The listing builds one solid part. Answer for the finished solid, in the listing's coordinates (mm). Face numbers are marked on the shaded views. A direction names the side the tool comes from. Coordinates: 2 decimals unless noted, no trailing zeros. Order: outer loops, then holes, each group sorted by start corner. A loop starts at its lowest first (then second) coordinate and runs counter-clockwise, first axis right, second up. Notation, with made-up numbers: (2, 42) -> (17, 42) arc R9 cw to (17, 50) -> close; hole circle Ø10 at (84, 17). An arc over 180 degrees is marked (long way). Write each question's results on one line, items separated by ' | '. Start each with the question number.
(1) Determine the mould class of the marked faces 1, 2 and 3 for opening direction X: +X half, -X half, draft (parallel to the pull), parting line (faces both ways), or undercut.
(2) The part is cut by section C-C, the plane z = -9. Count the separate pieces of the cut face and the enclosed holes in it, then the cut area to 3 significant figures.
(3) The part is cut by section B-B, the plane y = 9. Give the vertices of the cut face in (x, z), then the cut area to 3 significant figures.
(4) A tool of negligible diameter and unlimited length cuts with its end or side. For the marked faces 4 and 5, from which of +Z, -Z, +X, -X, +Y, -Y can it reach the whole face along a straight path? Write none if from no direction.
(5) The part is cut by section A-A, the plane x = 22. Give the vertices of the cut face in (y, z), then the cut area to 3 significant figures.
(6) Given pin 1 (10.5 mm diameter, centred on x = -37.69, z = 28.7, fed in from -Y); pin 2 (10.5 mm diameter, centred on x = -29.22, z = -27.5, fed in from +Y); pin 3 (5 mm diameter, centred on x = 9.56, z = 19.57, fed in from -Y); pin 4 (0.6 mm diameter, centred on x = -48, y = 7, fed in from +Z), each flat-ended and moving along its own axis, determine where each tip first touches the part or whether it passes through.
(7) Straight lines are drawn through the part: L1, parallel to X at y = 8.25, z = 23; L2, parallel to Y at x = 26.5, z = -26. For each, find the intervals that lie inside material, in ascending order.
```python
from build123d import *

# Parameters (mm, degrees)
SKETCH1_W               = 76.9234
SKETCH1_H               = 67.5
BASE_FLANGE1_DEPTH      = 0.7366
EDGE_FLANGE1_DEPTH      = 67.5
EDGE_FLANGE1_BEND_DEPTH = 67.5
CUT_EXTRUDE1_DEPTH      = 89.757105022
FILLET1_R               = 10
SKETCH14_R              = 4
CUT_EXTRUDE2_DEPTH      = 10


# Sheet-metal steps are written as plain solids
with BuildPart() as part:
    # Sketch1 → Base-Flange1 (new body)
    with BuildSketch(Plane(origin=(0, 0, 0), x_dir=(1, 0, 0), z_dir=(0, 1, 0))):
        with Locations((-8.2804, -1.046060421)):
            Rectangle(SKETCH1_W, SKETCH1_H)
    extrude(amount=-BASE_FLANGE1_DEPTH)

    # Edge-Flange1 section (across the edge) → Edge-Flange1 (add)
    with BuildSketch(Plane(origin=(31.1813, 0, 34.796060421), x_dir=(-1, 0, 0), z_dir=(0, 0, -1))):
        with BuildLine():
            Line((-0.7366, 0.7366), (-0.7366, 14.2634))
            Line((-0.7366, 14.2634), (0, 14.2634))
            Line((0, 14.2634), (0, 0.7366))
            ThreePointArc((0, 0.7366), (0.215745145, 0.215745145), (0.7366, 0))
            Line((0.7366, 0), (1, 0))
            Line((1, 0), (1, -0.7366))
            Line((1, -0.7366), (0.7366, -0.7366))
            ThreePointArc((0.7366, -0.7366), (-0.30510971, -0.30510971), (-0.7366, 0.7366))
        make_face()
    extrude(amount=EDGE_FLANGE1_DEPTH)

    # Edge-Flange1 section 2 (across the edge) → Edge-Flange1 bend (add)
    with BuildSketch(Plane(origin=(-47.7421, 0, -32.703939579), x_dir=(1, 0, 0), z_dir=(0, 0, 1))):
        with BuildLine():
            Line((-0.7366, 0.7366), (-0.7366, 14.2634))
            Line((-0.7366, 14.2634), (0, 14.2634))
            Line((0, 14.2634), (0, 0.7366))
            ThreePointArc((0, 0.7366), (0.215745145, 0.215745145), (0.7366, 0))
            Line((0.7366, 0), (1, 0))
            Line((1, 0), (1, -0.7366))
            Line((1, -0.7366), (0.7366, -0.7366))
            ThreePointArc((0.7366, -0.7366), (-0.30510971, -0.30510971), (-0.7366, 0.7366))
        make_face()
    extrude(amount=EDGE_FLANGE1_BEND_DEPTH)

    # Sketch13 → Cut-Extrude1 (cut, through all)
    with BuildSketch(Plane.ZY.offset(48.4787)):
        with BuildLine():
            Line((28.046060421, 11.2634), (28.046060421, 3.7634))
            ThreePointArc((28.046060421, 3.7634), (26.796060421, 2.5134), (25.546060421, 3.7634))
            Line((25.546060421, 3.7634), (25.546060421, 11.2634))
            ThreePointArc((25.546060421, 11.2634), (26.796060421, 12.5134), (28.046060421, 11.2634))
        make_face()
        with BuildLine():
            Line((-23.453939579, 11.2634), (-23.453939579, 3.7634))
            ThreePointArc((-23.453939579, 3.7634), (-24.703939579, 2.5134), (-25.953939579, 3.7634))
            Line((-25.953939579, 3.7634), (-25.953939579, 11.2634))
            ThreePointArc((-25.953939579, 11.2634), (-24.703939579, 12.5134), (-23.453939579, 11.2634))
        make_face()
    extrude(amount=-CUT_EXTRUDE1_DEPTH, mode=Mode.SUBTRACT)

    # Fillet1
    fillet1_edges = [part.edges().sort_by_distance(p)[0] for p in [
        (31.5496, 14.2634, 34.796060421),
        (31.5496, 14.2634, -32.703939579),
        (-48.1104, 14.2634, -32.703939579),
        (-48.1104, 14.2634, 34.796060421),
    ]]
    fillet(fillet1_edges, radius=FILLET1_R)

    # Sketch14 → Cut-Extrude2 (cut)
    with BuildSketch(Plane(origin=(0, 0, 0), x_dir=(1, 0, 0), z_dir=(0, 1, 0))):
        with Locations(Location((-10.107825022, 20.865751953, 0), (0, 0, 270))):
            Circle(SKETCH14_R)
        with Locations(Location((-10.107825022, 10.865751953, 0), (0, 0, 270))):
            Circle(SKETCH14_R)
        with Locations(Location((-9.205793222, -19.134248047, 0), (0, 0, 270))):
            Circle(SKETCH14_R)
        with Locations(Location((-9.205793222, -29.134248047, 0), (0, 0, 270))):
            Circle(SKETCH14_R)
        with Locations(Location((19.247878072, 26.50663709, 0), (0, 0, 270))):
            Circle(SKETCH14_R)
        with Locations(Location((19.247878072, 16.50663709, 0), (0, 0, 270))):
            Circle(SKETCH14_R)
        with Locations(Location((19.247878072, 6.50663709, 0), (0, 0, 270))):
            Circle(SKETCH14_R)
        with Locations(Location((19.247878072, -3.49336291, 0), (0, 0, 270))):
            Circle(SKETCH14_R)
        with Locations(Location((19.247878072, -13.49336291, 0), (0, 0, 270))):
            Circle(SKETCH14_R)
        with Locations(Location((19.247878072, -23.49336291, 0), (0, 0, 270))):
            Circle(SKETCH14_R)
        with Locations(Location((9.55786408, 20.430678866, 0), (0, 0, 270))):
            Circle(SKETCH14_R)
        with Locations(Location((9.55786408, 10.430678866, 0), (0, 0, 270))):
            Circle(SKETCH14_R)
        with Locations(Location((9.55786408, 0.430678866, 0), (0, 0, 270))):
            Circle(SKETCH14_R)
        with Locations(Location((9.55786408, -9.569321134, 0), (0, 0, 270))):
            Circle(SKETCH14_R)
        with Locations(Location((9.55786408, -19.569321134, 0), (0, 0, 270))):
            Circle(SKETCH14_R)
        with Locations(Location((9.55786408, -29.569321134, 0), (0, 0, 270))):
            Circle(SKETCH14_R)
        with Locations(Location((0.26115317, 26.362129758, 0), (0, 0, 270))):
            Circle(SKETCH14_R)
        with Locations(Location((0.26115317, 16.362129758, 0), (0, 0, 270))):
            Circle(SKETCH14_R)
        with Locations(Location((0.26115317, 6.362129758, 0), (0, 0, 270))):
            Circle(SKETCH14_R)
        with Locations(Location((0.26115317, -3.637870242, 0), (0, 0, 270))):
            Circle(SKETCH14_R)
        with Locations(Location((0.26115317, -13.637870242, 0), (0, 0, 270))):
            Circle(SKETCH14_R)
        with Locations(Location((0.26115317, -23.637870242, 0), (0, 0, 270))):
            Circle(SKETCH14_R)
        with Locations(Location((-19.91735253, 20.63989034, 0), (0, 0, 270))):
            Circle(SKETCH14_R)
        with Locations(Location((-19.91735253, 10.63989034, 0), (0, 0, 270))):
            Circle(SKETCH14_R)
        with Locations(Location((-19.91735253, 0.63989034, 0), (0, 0, 270))):
            Circle(SKETCH14_R)
        with Locations(Location((-19.91735253, -9.36010966, 0), (0, 0, 270))):
            Circle(SKETCH14_R)
        with Locations(Location((-19.91735253, -19.36010966, 0), (0, 0, 270))):
            Circle(SKETCH14_R)
        with Locations(Location((-19.91735253, -29.36010966, 0), (0, 0, 270))):
            Circle(SKETCH14_R)
        with Locations(Location((-29.215531727, 27.503898239, 0), (0, 0, 270))):
            Circle(SKETCH14_R)
        with Locations(Location((-29.215531727, 17.503898239, 0), (0, 0, 270))):
            Circle(SKETCH14_R)
        with Locations(Location((-29.215531727, 7.503898239, 0), (0, 0, 270))):
            Circle(SKETCH14_R)
        with Locations(Location((-29.215531727, -2.496101761, 0), (0, 0, 270))):
            Circle(SKETCH14_R)
        with Locations(Location((-29.215531727, -12.496101761, 0), (0, 0, 270))):
            Circle(SKETCH14_R)
        with Locations(Location((-29.215531727, -22.496101761, 0), (0, 0, 270))):
            Circle(SKETCH14_R)
        with Locations(Location((-37.689197421, 21.302640913, 0), (0, 0, 270))):
            Circle(SKETCH14_R)
        with Locations(Location((-37.689197421, 11.302640913, 0), (0, 0, 270))):
            Circle(SKETCH14_R)
        with Locations(Location((-37.689197421, 1.302640913, 0), (0, 0, 270))):
            Circle(SKETCH14_R)
        with Locations(Location((-37.689197421, -8.697359087, 0), (0, 0, 270))):
            Circle(SKETCH14_R)
        with Locations(Location((-37.689197421, -18.697359087, 0), (0, 0, 270))):
            Circle(SKETCH14_R)
        with Locations(Location((-37.689197421, -28.697359087, 0), (0, 0, 270))):
            Circle(SKETCH14_R)
    extrude(amount=-CUT_EXTRUDE2_DEPTH, mode=Mode.SUBTRACT)


solid = part.part
```
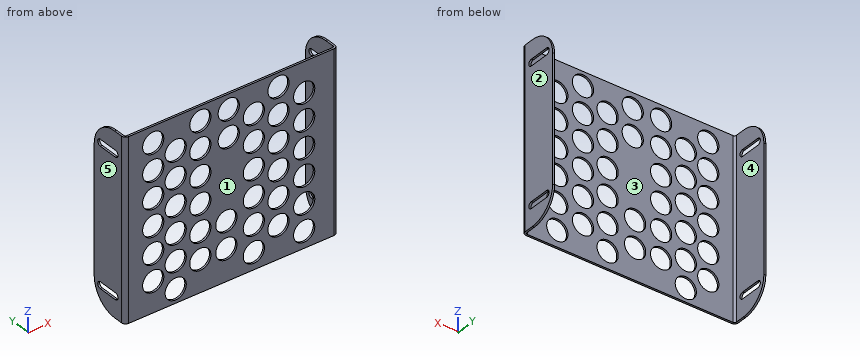
Established:
1) face 1: draft | face 2: +X half | face 3: undercut
2) separate pieces: 8 | enclosed holes: 0 | area: 44.1 mm^2
3) outline: (-48.48, -31.51) -> (-47.74, -31.51) -> (-47.74, -25.95) -> (-48.48, -25.95) -> close; (-48.48, -23.45) -> (-47.74, -23.45) -> (-47.74, 25.55) -> (-48.48, 25.55) -> close; (-48.48, 28.05) -> (-47.74, 28.05) -> (-47.74, 33.6) -> (-48.48, 33.6) -> close; (31.18, -31.51) -> (31.92, -31.51) -> (31.92, -25.95) -> (31.18, -25.95) -> close; (31.18, -23.45) -> (31.92, -23.45) -> (31.92, 25.55) -> (31.18, 25.55) -> close; (31.18, 28.05) -> (31.92, 28.05) -> (31.92, 33.6) -> (31.18, 33.6) -> close | area: 88.6 mm^2
4) face 4: +Z, -Z, +Y | face 5: +Z, -Z, -X, +Y, -Y
5) outline: (-0.74, -32.7) -> (0, -32.7) -> (0, -29.41) -> (-0.74, -29.41) -> close; (-0.74, -23.6) -> (0, -23.6) -> (0, -19.41) -> (-0.74, -19.41) -> close; (-0.74, -13.6) -> (0, -13.6) -> (0, -9.41) -> (-0.74, -9.41) -> close; (-0.74, -3.6) -> (0, -3.6) -> (0, 0.59) -> (-0.74, 0.59) -> close; (-0.74, 6.4) -> (0, 6.4) -> (0, 10.59) -> (-0.74, 10.59) -> close; (-0.74, 16.4) -> (0, 16.4) -> (0, 20.59) -> (-0.74, 20.59) -> close; (-0.74, 26.4) -> (0, 26.4) -> (0, 34.8) -> (-0.74, 34.8) -> close | area: 24.1 mm^2
6) pin 1: stops at y = -0.74 | pin 2: stops at y = 0 | pin 3: passes through | pin 4: stops at z = 34.49
7) L1: x = -48.48 to -47.74, 31.18 to 31.92 | L2: y = -0.74 to 0
